Check sheet for the modelled part. Datum: model origin and axes. Units: mm. Round coordinates to 2 decimals unless told otherwise and drop trailing zeros. Loops run counter-clockwise (first coordinate to the right, second up) from the corner with the lowest first, then second, coordinate; pieces in that order, holes last. Notation, with made-up numbers: (50, -30) - (80, -30) arc R13 ccw to (80, -8) - close; hole circle Ø8 at (77, -9). An arc over 180 degrees is marked (long way). Put each result on its own line as item: value.
```python
from build123d import *

# Parameters (mm, degrees)
SKETCH2_W                = 100
SKETCH2_H                = 110
BOSS_EXTRUDE1_DEPTH      = 8
SKETCH3_R                = 25
CUT_EXTRUDE1_DEPTH       = 9
SKETCH8_R                = 3
CUT_EXTRUDE2_DEPTH       = 9
F_9_0_9_DIAMETER_HOLE1_D = 9
M5X0_8_TAPPED_HOLE1_D    = 4.2
CHAMFER1_SIZE            = 3


with BuildPart() as part:
    # Sketch2 → Boss-Extrude1 (new body)
    with BuildSketch(Plane(origin=(0, 0, 0), x_dir=(0, 0, -1), z_dir=(1, 0, 0))):
        with Locations((0, 55)):
            Rectangle(SKETCH2_W, SKETCH2_H)
    extrude(amount=-BOSS_EXTRUDE1_DEPTH)

    # Sketch3 → Cut-Extrude1 (cut, through all)
    with BuildSketch(Plane(origin=(0, 0, 0), x_dir=(0, 0, -1), z_dir=(1, 0, 0))):
        with Locations((0, 55)):
            Circle(SKETCH3_R)
    extrude(amount=-CUT_EXTRUDE1_DEPTH, mode=Mode.SUBTRACT)

    # Sketch8 → Cut-Extrude2 (cut, through all)
    with BuildSketch(Plane.ZY.offset(8)):
        with Locations((0, 10)):
            Circle(SKETCH8_R)
        with Locations((0, 100)):
            Circle(SKETCH8_R)
    extrude(amount=-CUT_EXTRUDE2_DEPTH, mode=Mode.SUBTRACT)

    # Ø9.0 (9) Diameter Hole1 (through all)
    with Locations(Plane(origin=(0, 0, 0), x_dir=(0, 0, -1), z_dir=(1, 0, 0))):
        with Locations((-40, 100), (-40, 10), (40, 10), (40, 100)):
            Hole(F_9_0_9_DIAMETER_HOLE1_D / 2)

    # M5x0.8 Tapped Hole1 (through all)
    with Locations(Plane(origin=(0, 0, 0), x_dir=(0, 0, -1), z_dir=(1, 0, 0))):
        with Locations((24.748737342, 79.748737342), (-24.748737342, 79.748737342), (-24.748737342, 30.251262658), (24.748737342, 30.251262658)):
            Hole(M5X0_8_TAPPED_HOLE1_D / 2)

    # Chamfer1
    chamfer1_edges = [part.edges().sort_by_distance(p)[0] for p in [
        (-4, 0, -50),
        (-4, 0, 50),
        (-4, 110, 50),
        (-4, 110, -50),
    ]]
    chamfer(chamfer1_edges, length=CHAMFER1_SIZE)


solid = part.part
```
Item 1: Section check C-C on z = 40. Enter the section's corners in (x, y), then the cut area to 3 significant figures.
Filled sheet:
outline: (-8, 0) - (0, 0) - (0, 5.5) - (-8, 5.5) - close; (-8, 14.5) - (0, 14.5) - (0, 95.5) - (-8, 95.5) - close; (-8, 104.5) - (0, 104.5) - (0, 110) - (-8, 110) - close
area: 736 mm²
Item 2: Section check D-D on z = -7. Enter the section's corners in (x, y).
Filled sheet:
outline: (-8, 0) - (0, 0) - (0, 31) - (-8, 31) - close; (-8, 79) - (0, 79) - (0, 110) - (-8, 110) - close
Item 3: Thickness scan on line 1 (Y direction, x = -5.25, z = 0); line 2 (Y direction, x = -5.25, z = 40); line 3 (Z direction, x = -1.25, y = 9.5). Record the ranges inside material, lowest first. Write a range as from..to.
Filled sheet:
line 1: 0..7, 13..30, 80..97, 103..110
line 2: 0..5.5, 14.5..95.5, 104.5..110
line 3: -50..-44.47, -35.53..-2.96, 2.96..35.53, 44.47..50
Item 4: Section check A-A on y = 55. Enter the section's corners in (x, z), then the cut area to 3 significant figures.
Filled sheet:
outline: (-8, -50) - (0, -50) - (0, -25) - (-8, -25) - close; (-8, 25) - (0, 25) - (0, 50) - (-8, 50) - close
area: 400 mm²
Item 5: Go/stop test with flat-tipped pins: pin 1 (10.5 mm diameter, centred on y = 10, z = 40, fed in from -X); pin 2 (2.5 mm diameter, centred on y = 79.75, z = 24.75, fed in from -X). Record where each tip stops, or that it passes through.
Filled sheet:
pin 1: x = -8
pin 2: through
Item 6: Section check B-B on y = 100. Enter the section's corners in (x, z), then the cut area to 3 significant figures.
Filled sheet:
outline: (-8, -50) - (0, -50) - (0, -44.5) - (-8, -44.5) - close; (-8, -35.5) - (0, -35.5) - (0, -3) - (-8, -3) - close; (-8, 3) - (0, 3) - (0, 35.5) - (-8, 35.5) - close; (-8, 44.5) - (0, 44.5) - (0, 50) - (-8, 50) - close
area: 608 mm²
Item 7: Release check for a two-part mould opening along Z. For faces 1 (the flat face through (-4, 0, 1)), 2 (the flat face through (-4, 108, -49)), 3 (the flat face through (-4, 109, 48)), 4 (the cylindrical face through (-4, 10, -3)) record: +Z half, -Z half, draft (parallel to the pull), parting line (faces both ways), or undercut.
Filled sheet:
face 1: draft
face 2: -Z half
face 3: +Z half
face 4: undercut
